```python
from build123d import *

# Parameters (mm, degrees)
SKETCH1_R           = 12.5
BOSS_EXTRUDE1_DEPTH = 85
SKETCH2_W           = 8
SKETCH2_H           = 8
CUT_EXTRUDE1_DEPTH  = 80
CHAMFER1_SIZE       = 1.5


with BuildPart() as part:
    # Sketch1 → Boss-Extrude1 (new body)
    with BuildSketch(Plane.XY):
        Circle(SKETCH1_R)
    extrude(amount=BOSS_EXTRUDE1_DEPTH)

    # Sketch2 → Cut-Extrude1 (cut)
    with BuildSketch(Plane(origin=(0, 0, 0), x_dir=(-1, 0, 0), z_dir=(0, 0, -1))):
        with Locations((0, 12.5)):
            Rectangle(SKETCH2_W, SKETCH2_H)
    extrude(amount=-CUT_EXTRUDE1_DEPTH, mode=Mode.SUBTRACT)

    # Chamfer1
    chamfer1_edges = [part.edges().sort_by_distance(p)[0] for p in [
        (-7.288689869, -10.155048006, 0),
    ]]
    chamfer(chamfer1_edges, length=CHAMFER1_SIZE)


solid = part.part
```
Geometry: final body of the model. Coordinates: model frame, mm. A direction names the side the tool comes from. Round coordinates to 2 decimals unless told otherwise and drop trailing zeros. Order: outer loops, then holes, each group sorted by start corner. A loop starts at its lowest first (then second) coordinate and runs counter-clockwise, first axis right, second up. Notation, with made-up numbers: (-14.5, 42.5) - (30.5, 42.5) arc R18 ccw to (30.5, 75.5) - close; hole circle Ø5 at (-23, 27.25). An arc over 180 degrees is marked (long way). Use CSV: the item, a comma, the result in double quotes. Start each with the question number.
Q1. Access query for faces 4 (the face through (0, 8.5, 39)), 5 (the face through (-2.71, -12.203, 42.666)). Directions: +Z, -Z, +X, -X, +Y, -Y. A direction counts if a zero-diameter tool reaches every point of the face in a straight line with its end or side. Return the directions, or none.
Q2. Material intervals for line 1 along X through (y, z) = (0.25, 44); line 2 along Y through (x, z) = (-8, 38.5); line 3 along Y through (x, z) = (-4.75, 59.5), sorted ascending. Write a range as from..to.
Q3. Mould query, pull axis X, two halves, no side actions, for faces 1 (the face through (-4, 10, 39)), 2 (the face through (-0.44, -11.23, 0.24)), 3 (the face through (0, 0, 0)). Classes: +X half, -X half, draft (parallel to the pull), parting line (faces both ways), or undercut.
Q4. Section query A-A (x = 0). Return loops of the section in (y, z).
Q5. First-contact query: pin 1 (2 mm diameter, centred on x = 9.5, z = 32, fed in from +Y); pin 2 (1.5 mm diameter, centred on x = 7, z = 47.5, fed in from +Y); pin 3 (4 mm diameter, centred on x = -1.5, z = 42, fed in from +Y). Flat tips, straight axial feed; report the tip coordinate or a pass-through.
Q6. Section query B-B (z = 77.5). Return loops of the section in (x, y), and give its area (3 significant figures).
Result set:
1,face 4,"-Z, +Y"
1,face 5,"+Z, -Z"
2,line 1,"x = -12.5..12.5"
2,line 2,"y = -9.6..9.6"
2,line 3,"y = -11.56..11.56"
3,face 1,"undercut"
3,face 2,"parting line"
3,face 3,"draft"
4,outline,"(-12.5, 1.5) - (-11, 0) - (8.5, 0) - (8.5, 80) - (12.5, 80) - (12.5, 85) - (-12.5, 85) - close"
5,pin 1,"stops at y = 9.17"
5,pin 2,"stops at y = 10.83"
5,pin 3,"stops at y = 8.5"
6,outline,"(-4, 8.5) - (-4, 11.84) arc R12.5 ccw (long way) to (4, 11.84) - (4, 8.5) - close"
6,area,"461 mm2"
